Autodesk Inventor part; units mm, degrees
ref_plane "YZ Plane" through (0, 0, 0) normal (1, 0, 0) x (0, 1, 0)
ref_plane "XZ Plane" through (0, 0, 0) normal (0, 1, 0) x (-1, 0, 0)
ref_plane "XY Plane" through (0, 0, 0) normal (0, 0, 1) x (1, 0, 0)
sketch "Sketch1" plane through (0, 0, 0) normal (0, 0, 1) x (1, 0, 0)
  circle A0 centre (0, 0) radius 25.4
  line L0 (-33.02, -38.1) -> (33.02, -38.1)
  line L1 (33.02, -38.1) -> (33.02, 69.85)
  line L2 (33.02, 69.85) -> (-33.02, 69.85)
  line L3 (-33.02, 69.85) -> (-33.02, -38.1)
  dimension "d0" = 50.8
  dimension "d1" = 66.04
  dimension "d2" = 107.95
  dimension "d3" = 33.02
  dimension "d4" = 38.1
extrude "Extrusion1" add sketch "Sketch1" against normal blind 40.64
sketch "Sketch2" plane through (0, 0, -40.64) normal (0, 0, -1) x (-1, 0, 0)
  circle A0 centre (0, 0) radius 25.1006
extrude "Extrusion2" add sketch "Sketch2" against normal blind 12.7
sketch "Sketch3" plane through (-33.02, -38.1, 0) normal (0, -1, 0) x (1, 0, 0)
  line L0 (0, 0) -> (66.04, 0)
  line L1 (66.04, 0) -> (0, 0)
  line L2 (0, 0) -> (0, -95.25)
  line L3 (0, -95.25) -> (66.04, -95.25)
  line L4 (66.04, -95.25) -> (66.04, 0)
  line L5 (66.04, -40.64) -> (0, -40.64)
  arc A0 (0, -95.25) -> (66.04, -95.25) centre (33.02, -95.25) ccw
  line L6 (0, -40.64) -> (66.04, -40.64)
  line L7 (0, -40.64) -> (66.04, -40.64)
  line L8 (66.04, -40.64) -> (66.04, -95.25)
  line L9 (66.04, -95.25) -> (0, -95.25)
  line L10 (0, -95.25) -> (0, -40.64)
  point P0 (33.02, 0)
  dimension "d9" = 54.61
extrude "Extrusion3" add sketch "Sketch3" along normal mid plane 62.23 contours L5 L4 L3 L2 | L3 A0
sketch "Sketch4" plane through (-33.02, -38.1, 0) normal (0, -1, 0) x (1, 0, 0)
  point P0 (33.02, 0)
sketch "Sketch5" plane through (-33.02, -6.985, 0) normal (0, 1, 0) x (1, 0, 0)
  arc A0 (66.04, 95.25) -> (0, 95.25) centre (33.02, 95.25) ccw
  line L0 (66.04, 40.64) -> (66.04, 95.25)
  line L1 (0, 95.25) -> (66.04, 95.25)
  line L2 (66.04, 95.25) -> (66.04, 40.64)
  line L3 (66.04, 40.64) -> (0, 40.64)
  line L4 (0, 40.64) -> (0, 95.25)
  arc A1 (66.04, 95.25) -> (0, 95.25) centre (33.02, 95.25) ccw
  point P0 (33.02, 0)
extrude "Extrusion4" add sketch "Sketch5" along normal blind 123.19
sketch "Sketch6" plane through (-33.02, -69.215, 0) normal (0, -1, 0) x (1, 0, 0)
  arc A0 (0, -95.25) -> (66.04, -95.25) centre (33.02, -95.25) ccw
  line L0 (0, -95.25) -> (33.02, -95.25)
  circle A1 centre (33.02, -95.25) radius 26.67
  point P0 (33.02, 0)
  dimension "d16" = 53.34
extrude "Extrusion5" cut sketch "Sketch6" against normal blind 60.96
properties part number "Wrist1-lrg"
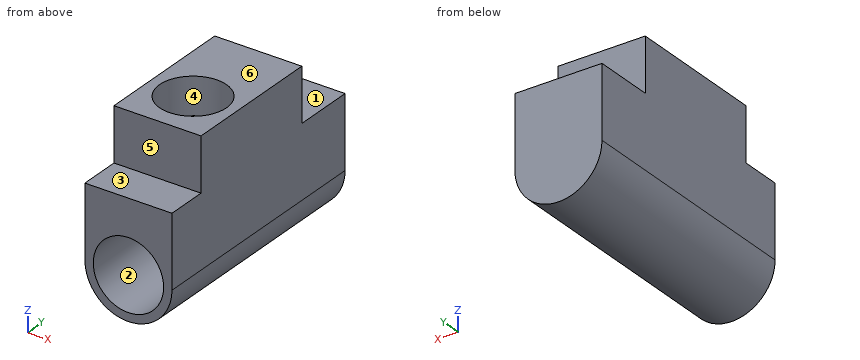
Check sheet for the modelled part. Datum: model origin and axes. Units: mm. Face numbers are marked on the shaded views. A direction names the side the tool comes from. Round coordinates to 2 decimals unless told otherwise and drop trailing zeros. Loops run counter-clockwise (first coordinate to the right, second up) from the corner with the lowest first, then second, coordinate; pieces in that order, holes last. Notation, with made-up numbers: M 23,-16 L 33,-16 A22 cw 33,11 Z; hole C 80,-10 d11. An arc over 180 degrees is marked long. One line per question, with ' | ' between items. Start each with the question number.
Item 1: Scan lines: probe 1 along X at (y, z) = (-33, -95.25); probe 2 along Z at (x, y) = (0, -53.5); probe 3 along Z at (x, y) = (0, -31). Record each from-to range of solid material in increasing order.
Item 2: Release check for a two-part mould opening along Y. For the marked faces 4, 5 and 6 record: released by +Y, released by -Y, zero draft, split by the parting line, or undercut.
Item 3: Set-up check for the marked faces 1, 2 and 3: record each of +Z, -Z, +X, -X, +Y, -Y from which the full face is reachable in a straight line by a thin tool's end or side.
Item 4: Section check C-C (x = 0). Record the boundary of the cut face in (y, z) (3 decimals), and give its area (3 significant figures).
Item 5: Section check D-D (y = -55.5). Record the boundary of the cut face in (x, z), and give its area (3 significant figures).
Item 6: Section check B-B (y = 0). Record the boundary of the cut face in (x, z), and give its area (3 significant figures).
Item 7: Gauge pin test, flat ends, axial feed: pin 1 Ø3 at (x, y) = (-17.5, -37) entering from -Z; pin 2 Ø12 at (x, z) = (-26, -21.5) entering from -Y; pin 3 Ø6 at (x, y) = (21, -45) entering from +Z. Record the tip position at first contact, or that the pin passes through.
Item 8: Section check A-A (z = -32.5). Record the boundary of the cut face in (x, y).
Worked out:
1) probe 1: -33.02 to -26.67, 26.67 to 33.02 | probe 2: -128.27 to -121.92, -68.58 to -40.64 | probe 3: -128.27 to -121.92, -68.58 to 0
2) face 4: undercut | face 5: released by -Y | face 6: zero draft
3) face 1: +Z, +X, -X, +Y | face 2: -Y | face 3: +Z, +X, -X, -Y
4) outline: M -69.215,-128.27 L 116.205,-128.27 L 116.205,-40.64 L 69.85,-40.64 L 69.85,0 L 25.4,0 L 25.4,-40.64 L 25.101,-40.64 L 25.101,-27.94 L -25.101,-27.94 L -25.101,-40.64 L -25.4,-40.64 L -25.4,0 L -38.1,0 L -38.1,-40.64 L -69.215,-40.64 L -69.215,-68.58 L -8.255,-68.58 L -8.255,-121.92 L -69.215,-121.92 Z | area: 16,000 mm^2
5) outline: M -33.02,-95.25 A33.02 ccw 33.02,-95.25 L 33.02,-40.64 L -33.02,-40.64 Z; hole C 0,-95.25 d53.34 | area: 3,080 mm^2
6) outline: M -33.02,-95.25 A33.02 ccw 33.02,-95.25 L 33.02,0 L 25.4,0 L 25.4,-40.64 L 25.1,-40.64 L 25.1,-27.94 L -25.1,-27.94 L -25.1,-40.64 L -25.4,-40.64 L -25.4,0 L -33.02,0 Z | area: 6,580 mm^2
7) pin 1: z = -124.13 | pin 2: y = -38.1 | pin 3: z = -40.64
8) outline: M -33.02,-38.1 L 33.02,-38.1 L 33.02,69.85 L -33.02,69.85 Z; C 0,0 d50.2; hole C 0,0 d50.8
